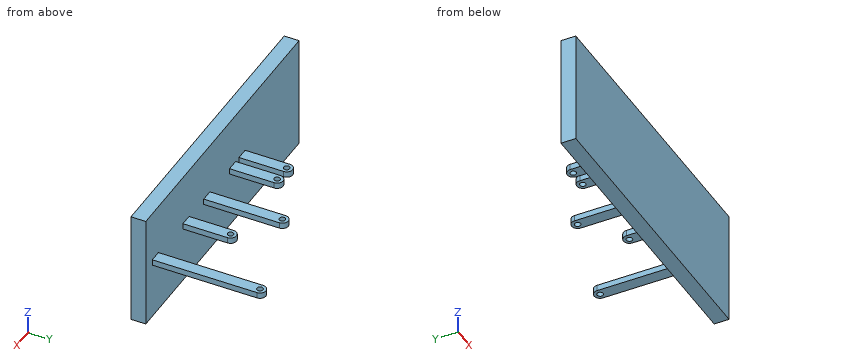
```python
from build123d import *

# Parameters (mm, degrees)
SKETCH_1_W      = 100
SKETCH_1_H      = 38.575985264
EXTRUDE_1_DEPTH = 5
SKETCH_2_R      = 1
EXTRUDE_2_DEPTH = 2


with BuildPart() as part:
    # 草圖1 → 填料-伸長1 (new body)
    with BuildSketch(Plane(origin=(0, 0, 0), x_dir=(1, 0, 0), z_dir=(0, 1, 0))):
        Rectangle(SKETCH_1_W, SKETCH_1_H)
    extrude(amount=EXTRUDE_1_DEPTH)

    # 草圖2 → 填料-伸長2 (add)
    # profile 1 of 5: a face of its own
    with BuildSketch(Plane.XY):
        with BuildLine():
            Line((-8.6, 20), (-8.6, 0))
            Line((-8.6, 0), (-4.6, 0))
            Line((-4.6, 0), (-4.6, 20))
            ThreePointArc((-4.6, 20), (-6.6, 22), (-8.6, 20))
        make_face()
        with Locations((-6.6, 20)):
            Circle(SKETCH_2_R, mode=Mode.SUBTRACT)
    # profile 2 of 5: a face of its own
    with BuildSketch(Plane.XY):
        with BuildLine():
            Line((-14.8, 20), (-14.8, 0))
            Line((-14.8, 0), (-10.8, 0))
            Line((-10.8, 0), (-10.8, 20))
            ThreePointArc((-10.8, 20), (-12.8, 22), (-14.8, 20))
        make_face()
        with Locations((-12.8, 20)):
            Circle(SKETCH_2_R, mode=Mode.SUBTRACT)
    # profile 3 of 5: a face of its own
    with BuildSketch(Plane.XY):
        with BuildLine():
            Line((21.8, 20), (21.8, 0))
            Line((21.8, 0), (25.8, 0))
            Line((25.8, 0), (25.8, 20))
            ThreePointArc((25.8, 20), (23.8, 22), (21.8, 20))
        make_face()
        with Locations((23.8, 20)):
            Circle(SKETCH_2_R, mode=Mode.SUBTRACT)
    # profile 4 of 5: a face of its own
    with BuildSketch(Plane.XY):
        with BuildLine():
            Line((8.2, 30.4), (8.2, 0))
            Line((8.2, 0), (12.2, 0))
            Line((12.2, 0), (12.2, 30.4))
            ThreePointArc((12.2, 30.4), (10.2, 32.4), (8.2, 30.4))
        make_face()
        with Locations((10.2, 30.4)):
            Circle(SKETCH_2_R, mode=Mode.SUBTRACT)
    # profile 5 of 5: a face of its own
    with BuildSketch(Plane.XY):
        with BuildLine():
            Line((41.78, 40.17), (41.78, 0))
            Line((41.78, 0), (45.78, 0))
            Line((45.78, 0), (45.78, 40.17))
            ThreePointArc((45.78, 40.17), (43.78, 42.17), (41.78, 40.17))
        make_face()
        with Locations((43.78, 40.17)):
            Circle(SKETCH_2_R, mode=Mode.SUBTRACT)
    extrude(amount=EXTRUDE_2_DEPTH)


solid = part.part
```
Verification items for the finished model (mm, model axes). Round coordinates to 2 decimals unless told otherwise and drop trailing zeros. Write each loop counter-clockwise with the first axis right and the second up, starting at its lowest first coordinate (ties: lowest second). Pieces come first, ordered by that corner, then holes. Notation, with made-up numbers: (25.5, -31.5) -> (35.5, -31.5) arc R29 cw to (35.5, 3.5) -> close; hole circle Ø8 at (53.5, 67.25). An arc over 180 degrees is marked (long way). Write each question's results on one line, items separated by ' | '. Start each with the question number.
1. Cross-section at B-B (y = 9.5). Enter the section's corners in (x, z), then the cut area to 3 significant figures.
2. Cross-section at A-A (x = -6.6). Enter the section's corners in (y, z), then the cut area to 3 significant figures.
3. Depth check by flat-ended pin: P1, Ø8, axis at x = -9.5, y = 20.5, coming from the +Z side; P2, Ø2, axis at x = 3, z = 1, coming from the -Y side; P3, Ø1, axis at y = 23.5, z = 1, coming from the +X side; P4, Ø8, axis at x = -39.5, z = -5.5, coming from the +Y side. Enter the tip coordinate at first touch or a pass-through.
4. Cross-section at C-C (x = 10.2). Enter the section's corners in (y, z).
5. Material ranges on probe 1 along Y at (x, z) = (-6.6, 1.6); probe 2 along Y at (x, z) = (43.78, 0.6); probe 3 along Y at (x, z) = (-43.5, 3.5), recorded low to high. Write a range as from..to.
6. Cross-section at D-D (z = -6). Enter the section's corners in (x, y), then the cut area to 3 significant figures.
Solutions:
1) outline: (-14.8, 0) -> (-10.8, 0) -> (-10.8, 2) -> (-14.8, 2) -> close; (-8.6, 0) -> (-4.6, 0) -> (-4.6, 2) -> (-8.6, 2) -> close; (8.2, 0) -> (12.2, 0) -> (12.2, 2) -> (8.2, 2) -> close; (21.8, 0) -> (25.8, 0) -> (25.8, 2) -> (21.8, 2) -> close; (41.78, 0) -> (45.78, 0) -> (45.78, 2) -> (41.78, 2) -> close | area: 40.0 mm2
2) outline: (0, -19.29) -> (5, -19.29) -> (5, 0) -> (19, 0) -> (19, 2) -> (5, 2) -> (5, 19.29) -> (0, 19.29) -> close; (21, 0) -> (22, 0) -> (22, 2) -> (21, 2) -> close | area: 223 mm2
3) P1: stops at z = 2 | P2: stops at y = 0 | P3: stops at x = 45.78 | P4: stops at y = 5
4) outline: (0, -19.29) -> (5, -19.29) -> (5, 0) -> (29.4, 0) -> (29.4, 2) -> (5, 2) -> (5, 19.29) -> (0, 19.29) -> close; (31.4, 0) -> (32.4, 0) -> (32.4, 2) -> (31.4, 2) -> close
5) probe 1: y = 0..19, 21..22 | probe 2: y = 0..39.17, 41.17..42.17 | probe 3: y = 0..5
6) outline: (-50, 0) -> (50, 0) -> (50, 5) -> (-50, 5) -> close | area: 500 mm2
